Design review of the part built by this model. Coordinates are the model's own, in mm. A direction names the side the tool comes from. Give positions to 0.01 mm unless a question says otherwise; leave off trailing zeros. Order: outer loops, then holes, each group sorted by start corner. A loop starts at its lowest first (then second) coordinate and runs counter-clockwise, first axis right, second up. Notation, with made-up numbers: (79.25, 63) -> (97.25, 63) arc R8 cw to (97.25, 73) -> close; hole circle Ø1 at (-27.5, -26). An arc over 180 degrees is marked (long way). One line per item, written item: value. Start each with the question number.
1) The part is to be moulded in two halves that separate along X. For faces 3 (the face through (42.607, -7.083, 7.513)), 4 (the face through (0, -39, 0)), 5 (the face through (32.103, 28.896, 7.513)), 6 (the face through (-58.386, 1.988, 7.513)), say which applies: released by +X, released by -X, zero draft, split by the parting line, or undercut.
2) Tool access review of faces 1 (the face through (254, -38.1, 8)), 2 (the face through (32.039, -28.754, 7.513)): name each direction out of +Z, -Z, +X, -X, +Y, -Y from which nothing blocks a thin tool from reaching the whole face with its end or side.
3) Consider section A-A (x = 362). State the section outline as (y, z) points, plus the area to 3 significant figures.
4) For pin 1 (1 mm diameter, centred on x = 131.5, z = 4.5, fed in from +Y); pin 2 (4 mm diameter, centred on x = 412.5, y = 0, fed in from +Z); pin 3 (8 mm diameter, centred on x = 336.5, z = 2.5, fed in from -Y), all flat-tipped, find the tip position at first contact; note any pin that passes through.
5) Wall thickness on line 1 along X through (y, z) = (42, 3.5); line 2 along Z through (x, y) = (95, 32.5); line 3 along X through (y, z) = (-16, 5.5): over which ranges is each line inside the solid? List them lowest first. Write a range as from..to.
from build123d import *

# Parameters (mm, degrees)
F0_R         = 58.42
F0_R_2       = 48.26
F1_DEPTH     = 15.24
F4_DEPTH     = 5.08
F6_DEPTH     = 7.62
F7_T4_ANGLE  = 67.8542971522
F7_T9_ANGLE  = 67.8542971522
F7_T14_ANGLE = 67.8542971522
F7_T19_ANGLE = 67.8542971522


# Not quite as in the source:
# - a fillet or chamfer that OpenCascade refuses, or shapes differently, is made with other operations: its cross-section is extruded or revolved along the edge and cut away or added


with BuildPart() as f1:
    # F0 (on Top) → F1 (new body)
    with BuildSketch(Plane.XY):
        Circle(F0_R)
        Circle(F0_R_2, mode=Mode.SUBTRACT)
    extrude(amount=F1_DEPTH)

    # F3 (on offset) → F4 (join, symmetric)
    with BuildSketch(Plane.XY.offset(7.62)):
        with BuildLine():
            Line((469.9, 38.1), (44.2864132664, 38.1))
            ThreePointArc((44.2864132664, 38.1), (58.3891573479, 0), (44.2864132664, -38.1))
            Line((44.2864132664, -38.1), (469.9, -38.1))
            ThreePointArc((469.9, -38.1), (508, 0), (469.9, 38.1))
        make_face()
    extrude(amount=F4_DEPTH, both=True)

    # F5 (on offset) → F6 (join, symmetric)
    with BuildSketch(Plane.XY.offset(7.62)):
        with BuildLine():
            Line((-15.6318332701, 45.6582236691), (-8.4780475837, 37.1447534541))
            Line((-8.4780475837, 37.1447534541), (-5.7265656824, 47.9190363581))
            ThreePointArc((-5.7265656824, 47.9190363581), (-10.7388602727, 47.0500210419), (-15.6318332701, 45.6582236691))
        make_face()
        with BuildLine():
            Line((-5.08, 47.9918868143), (0, 38.1))
            Line((0, 38.1), (5.08, 47.9918868143))
            ThreePointArc((5.08, 47.9918868143), (0, 48.26), (-5.08, 47.9918868143))
        make_face()
        with BuildLine():
            Line((5.7265656824, 47.9190363581), (8.4780475837, 37.1447534541))
            Line((8.4780475837, 37.1447534541), (15.6318332701, 45.6582236691))
            ThreePointArc((15.6318332701, 45.6582236691), (10.7388602727, 47.0500210419), (5.7265656824, 47.9190363581))
        make_face()
        with BuildLine():
            Line((16.2459774494, 45.4433253263), (16.5309704604, 34.3269138671))
            Line((16.5309704604, 34.3269138671), (25.3998211473, 41.0350665369))
            ThreePointArc((25.3998211473, 41.0350665369), (20.9392292498, 43.480757565), (16.2459774494, 45.4433253263))
        make_face()
        with BuildLine():
            Line((25.9507480698, 40.6888962079), (23.7549614508, 29.787779482))
            Line((23.7549614508, 29.787779482), (33.8941559316, 34.354239821))
            ThreePointArc((33.8941559316, 34.354239821), (30.0896178377, 37.7311873439), (25.9507480698, 40.6888962079))
        make_face()
        with BuildLine():
            Line((34.354239821, 33.8941559316), (29.787779482, 23.7549614508))
            Line((29.787779482, 23.7549614508), (40.6888962079, 25.9507480698))
            ThreePointArc((40.6888962079, 25.9507480698), (37.7311873439, 30.0896178377), (34.354239821, 33.8941559316))
        make_face()
        with BuildLine():
            Line((41.0350665369, 25.3998211473), (34.3269138671, 16.5309704604))
            Line((34.3269138671, 16.5309704604), (45.4433253263, 16.2459774494))
            ThreePointArc((45.4433253263, 16.2459774494), (43.480757565, 20.9392292498), (41.0350665369, 25.3998211473))
        make_face()
        with BuildLine():
            Line((45.6582236691, 15.6318332701), (37.1447534541, 8.4780475837))
            Line((37.1447534541, 8.4780475837), (47.9190363581, 5.7265656824))
            ThreePointArc((47.9190363581, 5.7265656824), (47.0500210419, 10.7388602727), (45.6582236691, 15.6318332701))
        make_face()
        with BuildLine():
            Line((47.9918868143, 5.08), (38.1, 0))
            Line((38.1, 0), (47.9918868143, -5.08))
            ThreePointArc((47.9918868143, -5.08), (48.26, 0), (47.9918868143, 5.08))
        make_face()
        with BuildLine():
            Line((47.9190363581, -5.7265656824), (37.1447534541, -8.4780475837))
            Line((37.1447534541, -8.4780475837), (45.6582236691, -15.6318332701))
            ThreePointArc((45.6582236691, -15.6318332701), (47.0500210419, -10.7388602727), (47.9190363581, -5.7265656824))
        make_face()
        with BuildLine():
            Line((45.4433253263, -16.2459774494), (34.3269138671, -16.5309704604))
            Line((34.3269138671, -16.5309704604), (41.0350665369, -25.3998211473))
            ThreePointArc((41.0350665369, -25.3998211473), (43.480757565, -20.9392292498), (45.4433253263, -16.2459774494))
        make_face()
        with BuildLine():
            Line((40.6888962079, -25.9507480698), (29.787779482, -23.7549614508))
            Line((29.787779482, -23.7549614508), (34.354239821, -33.8941559316))
            ThreePointArc((34.354239821, -33.8941559316), (37.7311873439, -30.0896178377), (40.6888962079, -25.9507480698))
        make_face()
        with BuildLine():
            Line((25.3998211473, -41.0350665369), (16.5309704604, -34.3269138671))
            Line((16.5309704604, -34.3269138671), (16.2459774494, -45.4433253263))
            ThreePointArc((16.2459774494, -45.4433253263), (20.9392292498, -43.480757565), (25.3998211473, -41.0350665369))
        make_face()
        with BuildLine():
            Line((15.6318332701, -45.6582236691), (8.4780475837, -37.1447534541))
            Line((8.4780475837, -37.1447534541), (5.7265656824, -47.9190363581))
            ThreePointArc((5.7265656824, -47.9190363581), (10.7388602727, -47.0500210419), (15.6318332701, -45.6582236691))
        make_face()
        with BuildLine():
            Line((5.08, -47.9918868143), (0, -38.1))
            Line((0, -38.1), (-5.08, -47.9918868143))
            ThreePointArc((-5.08, -47.9918868143), (0, -48.26), (5.08, -47.9918868143))
        make_face()
        with BuildLine():
            Line((33.8941559316, -34.354239821), (23.7549614508, -29.787779482))
            Line((23.7549614508, -29.787779482), (25.9507480698, -40.6888962079))
            ThreePointArc((25.9507480698, -40.6888962079), (30.0896178377, -37.7311873439), (33.8941559316, -34.354239821))
        make_face()
        with BuildLine():
            Line((-5.7265656824, -47.9190363581), (-8.4780475837, -37.1447534541))
            Line((-8.4780475837, -37.1447534541), (-15.6318332701, -45.6582236691))
            ThreePointArc((-15.6318332701, -45.6582236691), (-10.7388602727, -47.0500210419), (-5.7265656824, -47.9190363581))
        make_face()
        with BuildLine():
            Line((-16.2459774494, -45.4433253263), (-16.5309704604, -34.3269138671))
            Line((-16.5309704604, -34.3269138671), (-25.3998211473, -41.0350665369))
            ThreePointArc((-25.3998211473, -41.0350665369), (-20.9392292498, -43.480757565), (-16.2459774494, -45.4433253263))
        make_face()
        with BuildLine():
            Line((-25.9507480698, -40.6888962079), (-23.7549614508, -29.787779482))
            Line((-23.7549614508, -29.787779482), (-33.8941559316, -34.354239821))
            ThreePointArc((-33.8941559316, -34.354239821), (-30.0896178377, -37.7311873439), (-25.9507480698, -40.6888962079))
        make_face()
        with BuildLine():
            Line((-34.354239821, -33.8941559316), (-29.787779482, -23.7549614508))
            Line((-29.787779482, -23.7549614508), (-40.6888962079, -25.9507480698))
            ThreePointArc((-40.6888962079, -25.9507480698), (-37.7311873439, -30.0896178377), (-34.354239821, -33.8941559316))
        make_face()
        with BuildLine():
            Line((-41.0350665369, -25.3998211473), (-34.3269138671, -16.5309704604))
            Line((-34.3269138671, -16.5309704604), (-45.4433253263, -16.2459774494))
            ThreePointArc((-45.4433253263, -16.2459774494), (-43.480757565, -20.9392292498), (-41.0350665369, -25.3998211473))
        make_face()
        with BuildLine():
            Line((-45.6582236691, -15.6318332701), (-37.1447534541, -8.4780475837))
            Line((-37.1447534541, -8.4780475837), (-47.9190363581, -5.7265656824))
            ThreePointArc((-47.9190363581, -5.7265656824), (-47.0500210419, -10.7388602727), (-45.6582236691, -15.6318332701))
        make_face()
        with BuildLine():
            Line((-47.9918868143, -5.08), (-38.1, 0))
            Line((-38.1, 0), (-47.9918868143, 5.08))
            ThreePointArc((-47.9918868143, 5.08), (-48.26, 0), (-47.9918868143, -5.08))
        make_face()
        with BuildLine():
            Line((-47.9190363581, 5.7265656824), (-37.1447534541, 8.4780475837))
            Line((-37.1447534541, 8.4780475837), (-45.6582236691, 15.6318332701))
            ThreePointArc((-45.6582236691, 15.6318332701), (-47.0500210419, 10.7388602727), (-47.9190363581, 5.7265656824))
        make_face()
        with BuildLine():
            Line((-45.4433253263, 16.2459774494), (-34.3269138671, 16.5309704604))
            Line((-34.3269138671, 16.5309704604), (-41.0350665369, 25.3998211473))
            ThreePointArc((-41.0350665369, 25.3998211473), (-43.480757565, 20.9392292498), (-45.4433253263, 16.2459774494))
        make_face()
        with BuildLine():
            Line((-40.6888962079, 25.9507480698), (-29.787779482, 23.7549614508))
            Line((-29.787779482, 23.7549614508), (-34.354239821, 33.8941559316))
            ThreePointArc((-34.354239821, 33.8941559316), (-37.7311873439, 30.0896178377), (-40.6888962079, 25.9507480698))
        make_face()
        with BuildLine():
            Line((-33.8941559316, 34.354239821), (-23.7549614508, 29.787779482))
            Line((-23.7549614508, 29.787779482), (-25.9507480698, 40.6888962079))
            ThreePointArc((-25.9507480698, 40.6888962079), (-30.0896178377, 37.7311873439), (-33.8941559316, 34.354239821))
        make_face()
        with BuildLine():
            Line((-25.3998211473, 41.0350665369), (-16.5309704604, 34.3269138671))
            Line((-16.5309704604, 34.3269138671), (-16.2459774494, 45.4433253263))
            ThreePointArc((-16.2459774494, 45.4433253263), (-20.9392292498, 43.480757565), (-25.3998211473, 41.0350665369))
        make_face()
    extrude(amount=F6_DEPTH, both=True)

    # F7: fillet of radius 25.4 on 4 edges, made by hand


with BuildPart() as f7_tool2:
    # F7_s3 → F7_t4 (revolve)
    with BuildSketch(Plane.XZ):
        with BuildLine():
            ThreePointArc((58.42, 15.24), (63.8119906537, 13.3431423642), (69.4916033166, 12.7))
            Line((69.4916033166, 12.7), (58.42, 12.7))
            Line((58.42, 12.7), (58.42, 15.24))
        make_face()
    revolve(axis=Axis((0, 0, 12.7), (0, 0, -1)), revolution_arc=F7_T4_ANGLE)

    split(bisect_by=Plane.XZ.offset(38.1), keep=Keep.BOTTOM)


with BuildPart() as f1_1:
    add(f1.part)

    # F7_t1: union F7_tool2
    add(f7_tool2.part)


with BuildPart() as f7_tool7:
    # F7_s8 → F7_t9 (revolve)
    with BuildSketch(Plane(origin=(0, 0, 0), x_dir=(0, 0, 1), z_dir=(-0.9262282352, 0.376963203, 0))):
        with BuildLine():
            ThreePointArc((15.24, 58.42), (13.3431423642, 63.8119906537), (12.7, 69.4916033166))
            Line((12.7, 69.4916033166), (12.7, 58.42))
            Line((12.7, 58.42), (15.24, 58.42))
        make_face()
    revolve(axis=Axis((0, 0, 12.7), (0, 0, -1)), revolution_arc=F7_T9_ANGLE)

    split(bisect_by=Plane.XZ.offset(-38.1), keep=Keep.TOP)


with BuildPart() as f1_2:
    add(f1_1.part)

    # F7_t6: union F7_tool7
    add(f7_tool7.part)


with BuildPart() as f7_tool12:
    # F7_s13 → F7_t14 (revolve)
    with BuildSketch(Plane.XZ):
        with BuildLine():
            ThreePointArc((58.42, 0), (63.8119906537, 1.8968576358), (69.4916033166, 2.54))
            Line((69.4916033166, 2.54), (58.42, 2.54))
            Line((58.42, 2.54), (58.42, 0))
        make_face()
    revolve(axis=Axis((0, 0, 2.54), (0, 0, -1)), revolution_arc=F7_T14_ANGLE)

    split(bisect_by=Plane.XZ.offset(38.1), keep=Keep.BOTTOM)


with BuildPart() as f1_3:
    add(f1_2.part)

    # F7_t11: union F7_tool12
    add(f7_tool12.part)


with BuildPart() as f7_tool17:
    # F7_s18 → F7_t19 (revolve)
    with BuildSketch(Plane(origin=(0, 0, 0), x_dir=(0, 0, 1), z_dir=(-0.9262282352, 0.376963203, 0))):
        with BuildLine():
            ThreePointArc((0, 58.42), (1.8968576358, 63.8119906537), (2.54, 69.4916033166))
            Line((2.54, 69.4916033166), (2.54, 58.42))
            Line((2.54, 58.42), (0, 58.42))
        make_face()
    revolve(axis=Axis((0, 0, 2.54), (0, 0, -1)), revolution_arc=F7_T19_ANGLE)

    split(bisect_by=Plane.XZ.offset(-38.1), keep=Keep.TOP)


with BuildPart() as f1_4:
    add(f1_3.part)

    # F7_t16: union F7_tool17
    add(f7_tool17.part)


solid = f1_4.part
Checked values:
1. face 3: undercut
1. face 4: zero draft
1. face 5: undercut
1. face 6: split by the parting line
2. face 1: +Z, -Z, +X, -Y
2. face 2: +Z, -Z
3. outline: (-38.1, 2.54) -> (38.1, 2.54) -> (38.1, 12.7) -> (-38.1, 12.7) -> close
3. area: 774 mm^2
4. pin 1: stops at y = 38.1
4. pin 2: stops at z = 12.7
4. pin 3: stops at y = -38.1
5. line 1: x = -40.61..-16.33, -12.56..-7.24, -2..2, 7.24..12.56, 16.33..40.61
5. line 2: z = 2.54..12.7
5. line 3: x = -56.19..-45.53, 45.53..504.48
